```python
from build123d import *

# Parameters (mm, degrees)
SKETCH1_R           = 3.175
SKETCH1_R_2         = 2.7
SKETCH1_R_3         = 14
BOSS_EXTRUDE1_DEPTH = 4.7625
FILLET1_R           = 15.24


with BuildPart() as part:
    # Sketch1 → Boss-Extrude1 (new body)
    with BuildSketch(Plane(origin=(0, 0, 0), x_dir=(1, 0, 0), z_dir=(0, 1, 0))):
        with BuildLine():
            Line((114.3, 20.32), (0, 20.32))
            ThreePointArc((0, 20.32), (-14.368409794, 14.368409794), (-20.32, 0))
            Line((-20.32, 0), (-20.32, -172.72))
            Line((-20.32, -172.72), (114.3, -172.72))
            Line((114.3, -172.72), (114.3, 20.32))
        make_face()
        with Locations(Location((-6.604, -152.4, 0), (0, 0, 90))):
            Circle(SKETCH1_R, mode=Mode.SUBTRACT)
        with Locations(Location((29.297861909, -127.72, 0), (0, 0, 90))):
            Circle(SKETCH1_R_2, mode=Mode.SUBTRACT)
        with Locations(Location((29.297861909, -87.72, 0), (0, 0, 90))):
            Circle(SKETCH1_R_2, mode=Mode.SUBTRACT)
        with Locations(Location((96.52, -152.4, 0), (0, 0, 90))):
            Circle(SKETCH1_R, mode=Mode.SUBTRACT)
        with Locations(Location((89.297861909, -127.72, 0), (0, 0, 90))):
            Circle(SKETCH1_R_2, mode=Mode.SUBTRACT)
        with Locations(Location((89.297861909, -87.72, 0), (0, 0, 90))):
            Circle(SKETCH1_R_2, mode=Mode.SUBTRACT)
        with Locations(Location((29.297861909, -47.72, 0), (0, 0, 90))):
            Circle(SKETCH1_R_2, mode=Mode.SUBTRACT)
        with Locations(Location((-6.604, -25.4, 0), (0, 0, 90))):
            Circle(SKETCH1_R, mode=Mode.SUBTRACT)
        with Locations(Location((89.297861909, -47.72, 0), (0, 0, 90))):
            Circle(SKETCH1_R_2, mode=Mode.SUBTRACT)
        with Locations(Location((52.07, 6.604, 0), (0, 0, 90))):
            Circle(SKETCH1_R, mode=Mode.SUBTRACT)
        with Locations(Location((102.87, 6.604, 0), (0, 0, 90))):
            Circle(SKETCH1_R, mode=Mode.SUBTRACT)
        with Locations(Location((0, 0, 0), (0, 0, 90))):
            Circle(SKETCH1_R_3, mode=Mode.SUBTRACT)
    extrude(amount=BOSS_EXTRUDE1_DEPTH)

    # Fillet1
    fillet1_edges = [part.edges().sort_by_distance(p)[0] for p in [
        (114.3, 2.38125, -20.32),
        (114.3, 2.38125, 172.72),
        (-20.32, 2.38125, 172.72),
    ]]
    fillet(fillet1_edges, radius=FILLET1_R)


solid = part.part
```
Geometry: final body of the model. Coordinates: model frame, mm. Round coordinates to 2 decimals unless told otherwise and drop trailing zeros. Loops run counter-clockwise (first coordinate to the right, second up) from the corner with the lowest first, then second, coordinate; pieces in that order, holes last.
Item 1: Mould query, pull axis X, two halves, no side actions, for faces 1 (the cylindrical face through (105.97, 2.35, -5.92)), 2 (the flat face through (46, 0, 75)), 3 (the cylindrical face through (-15.74, 2.41, 168.37)). Classes: released by +X, released by -X, zero draft, split by the parting line, or undercut.
Checked values:
face 1: undercut
face 2: zero draft
face 3: released by -X
Item 2: Contact query for a flat-ended pin moving along its axis: P1, Ø17, axis at x = 0, z = 0, coming from the +Y side. Output: stop coordinate, or through.
Checked values:
P1: passes through
Item 3: Section C-C, the plane y = 1.15. State how many separate pieces and enclosed holes the cut face has, plus the area to 3 significant figures.
Checked values:
separate pieces: 1
enclosed holes: 12
area: 24,800 mm2
Item 4: Section D-D, the plane x = 11. Output: boundary loops of the cut face in (y, z).
Checked values:
outline: (0, -20.32) - (4.76, -20.32) - (4.76, -8.66) - (0, -8.66) - close; (0, 8.66) - (4.76, 8.66) - (4.76, 172.72) - (0, 172.72) - close
Item 5: Section B-B, the plane x = 96.52. Output: boundary loops of the cut face in (y, z) (1 decimal).
Checked values:
outline: (0, -20.3) - (4.8, -20.3) - (4.8, 149.2) - (0, 149.2) - close; (0, 155.6) - (4.8, 155.6) - (4.8, 172.7) - (0, 172.7) - close
Item 6: Section A-A, the plane z = 47.72. Output: boundary loops of the cut face in (x, y), plus the area to 3 significant figures.
Checked values:
outline: (-20.32, 0) - (26.6, 0) - (26.6, 4.76) - (-20.32, 4.76) - close; (32, 0) - (86.6, 0) - (86.6, 4.76) - (32, 4.76) - close; (92, 0) - (114.3, 0) - (114.3, 4.76) - (92, 4.76) - close
area: 590 mm2
Item 7: Line query: L1, parallel to X at y = 1.3, z = 152.4 (3 decimals); L2, parallel to Z at x = 28.5, y = 0.45; L3, parallel to X at y = 2.5, z = 127.72. Output: solid intervals per line, ascending.
Checked values:
L1: x = -20.32 to -9.779, -3.429 to 93.345, 99.695 to 114.3
L2: z = -20.32 to 45.14, 50.3 to 85.14, 90.3 to 125.14, 130.3 to 172.72
L3: x = -20.32 to 26.6, 32 to 86.6, 92 to 114.3
